Here's how the part is built. I have some questions about the finished solid (model axes, mm). Face numbers are marked on the shaded views. Coordinates: 2 decimals unless noted, no trailing zeros. Write each loop counter-clockwise with the first axis right and the second up, starting at its lowest first coordinate (ties: lowest second). Pieces come first, ordered by that corner, then holes. Notation, with made-up numbers: (74, 83) -> (117, 83) arc R30 cw to (117, 116) -> close; hole circle Ø10 at (49, -31.75). An arc over 180 degrees is marked (long way). Use a Markdown table: item, result. Add a question column.
Item 1: Will these pins go through, and if not, where does the flat tip stop? pin 1 Ø3 at (x, z) = (4, 1.5) entering from -Y; pin 2 Ø1 at (y, z) = (0.5, 7) entering from -X; pin 3 Ø3.5 at (x, z) = (0, 0) entering from +Y; pin 4 Ø1 at (x, y) = (-6, 2) entering from -Z.
Item 2: If we mould it in two halves opening along Z, with no side actions, what happens to the marked faces 1, 2, 3 and 4? For each: pulls with the +Z half, pulls with the -Z half, needs draft (parallel to the pull), parting line crosses it, or undercut.
Item 3: If I drill on line 1 along Z through (x, y) = (0, 1.25); line 2 along X through (y, z) = (1.2, 10); line 3 along Z through (x, y) = (1, 1.55), over which ranges is the centre line in solid material (lowest first)? Write a range as from..to.
Item 4: Imagine slicing it at B-B, the plane x = 0. Write out the boundary of the cut face in (y, z).
Item 5: Imagine slicing it at C-C, the plane x = -4.5. Write out the boundary of the cut face in (y, z) (3 decimals), and give its area (3 significant figures).
Item 6: Imagine slicing it at D-D, the plane y = 2.3. Count the separate pieces of the cut face and the enclosed holes in it, and give its area (3 significant figures).
Item 7: Imagine slicing it at A-A, the plane z = 0. Write out the boundary of the cut face in (x, y).
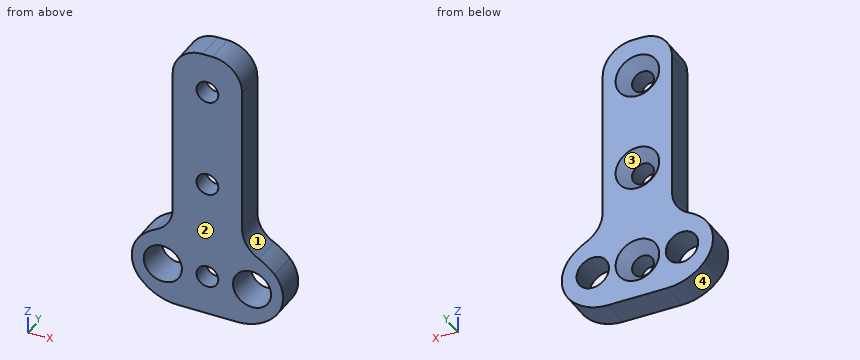
```python
from build123d import *

# Parameters (mm, degrees)
BOSS_EXTRUDE1_DEPTH                                 = 3
CSK_FOR_M2_COUNTERSUNK_FLAT_HEAD_SCREW3_D           = 2.2
CSK_FOR_M2_COUNTERSUNK_FLAT_HEAD_SCREW3_DEPTH       = 3
CSK_FOR_M2_COUNTERSUNK_FLAT_HEAD_SCREW3_CSINK_D     = 4.4
CSK_FOR_M2_COUNTERSUNK_FLAT_HEAD_SCREW3_CSINK_ANGLE = 90
CSK_FOR_M2_COUNTERSUNK_FLAT_HEAD_SCREW3_TIP         = 0.660946681
FILLET1_R                                           = 5
FILLET2_R                                           = 3.5
FILLET3_R                                           = 3
CSK_FOR_M2_COUNTERSUNK_FLAT_HEAD_SCR_2_COUNT        = 2
CSK_FOR_M2_COUNTERSUNK_FLAT_HEAD_SCR_2_PITCH        = 9


with BuildPart() as part:
    # Sketch1 → Boss-Extrude1 (new body)
    with BuildSketch(Plane(origin=(0, 0, 0), x_dir=(1, 0, 0), z_dir=(0, 1, 0))):
        Polygon((3.5, 6), (8, 6), (8, 14), (-8, 14), (-8, 6), (-3.5, 6), (-3.5, -14), (3.5, -14), align=None)
    extrude(amount=BOSS_EXTRUDE1_DEPTH)

    # CSK for M2 Countersunk Flat Head Screw3
    with Locations(Plane(origin=(0, 3, 0), x_dir=(1, 0, 0), z_dir=(0, 1, 0))):
        with Locations((0, 10), (0, 0), (0, -10)):
            CounterSinkHole(CSK_FOR_M2_COUNTERSUNK_FLAT_HEAD_SCREW3_D / 2, CSK_FOR_M2_COUNTERSUNK_FLAT_HEAD_SCREW3_CSINK_D / 2, depth=CSK_FOR_M2_COUNTERSUNK_FLAT_HEAD_SCREW3_DEPTH, counter_sink_angle=CSK_FOR_M2_COUNTERSUNK_FLAT_HEAD_SCREW3_CSINK_ANGLE)
            with Locations((0, 0, -(CSK_FOR_M2_COUNTERSUNK_FLAT_HEAD_SCREW3_DEPTH + CSK_FOR_M2_COUNTERSUNK_FLAT_HEAD_SCREW3_TIP / 2))):  # 118° drill point
                Cone(0, CSK_FOR_M2_COUNTERSUNK_FLAT_HEAD_SCREW3_D / 2, CSK_FOR_M2_COUNTERSUNK_FLAT_HEAD_SCREW3_TIP, mode=Mode.SUBTRACT)

    # Fillet1
    # the kernel refuses this fillet: 5 mm, written as the material it takes off along each edge
    with BuildSketch(Plane(origin=(-8, -12.437342964, -6), x_dir=(1, 0, 0), z_dir=(0, 1, 0))) as fillet1_piece_1:
        with BuildLine():
            CenterArc((5, 4.974937186), FILLET1_R, 180, 84.260829523)
            Line((0, 4.974937186), (-0.1, 4.974937186))
            Line((-0.1, 4.974937186), (-0.1, 0))
            Line((-0.1, 0), (0, -0.1))
            ThreePointArc((0, -0.1), (2.25, -0.1), (4.49, -0.099498744))
            Line((4.49, -0.099498744), (4.5, 0))
        make_face()
    extrude(amount=27.874685928, mode=Mode.SUBTRACT)
    with BuildSketch(Plane(origin=(-8, -12.5, -14), x_dir=(0, 0, 1), z_dir=(0, 1, 0)), Plane(origin=(8, -12.5, -14), x_dir=(-1, 0, 0), z_dir=(0, 1, 0))) as fillet1_piece_2:
        with BuildLine():
            CenterArc((FILLET1_R, FILLET1_R), FILLET1_R, 180, 90)
            Line((0, FILLET1_R), (-FILLET1_R * 0.02, FILLET1_R))
            Line((-FILLET1_R * 0.02, FILLET1_R), (-FILLET1_R * 0.02, -FILLET1_R * 0.02))
            Line((-FILLET1_R * 0.02, -FILLET1_R * 0.02), (FILLET1_R, -FILLET1_R * 0.02))
            Line((FILLET1_R, -FILLET1_R * 0.02), (FILLET1_R, 0))
        make_face()
    extrude(amount=28, mode=Mode.SUBTRACT)
    with BuildSketch(Plane(origin=(8, -12.437342964, -6), x_dir=(-1, 0, 0), z_dir=(0, 1, 0))) as fillet1_piece_3:
        with BuildLine():
            CenterArc((5, -4.974937186), FILLET1_R, 95.739170477, 84.260829523)
            Line((0, -4.974937186), (-0.1, -4.974937186))
            Line((-0.1, -4.974937186), (-0.1, 0))
            Line((-0.1, 0), (0, 0.1))
            ThreePointArc((0, 0.1), (2.25, 0.1), (4.49, 0.099498744))
            Line((4.49, 0.099498744), (4.5, 0))
        make_face()
    extrude(amount=27.874685928, mode=Mode.SUBTRACT)

    # Fillet2
    fillet2_edges = [part.edges().sort_by_distance(p)[0] for p in [
        (-7.901520762, 1.5, -9.987468593),
        (7.901520762, 1.5, -9.987468593),
    ]]
    fillet(fillet2_edges, radius=FILLET2_R)

    # Fillet3
    fillet3_edges = [part.edges().sort_by_distance(p)[0] for p in [
        (3.5, 1.5, -6),
        (3.5, 1.5, 14),
        (-3.5, 1.5, 14),
        (-3.5, 1.5, -6),
    ]]
    fillet(fillet3_edges, radius=FILLET3_R)

    # Sketch8 → CSK for M2 Countersunk Flat Head Screw2 (revolve, cut)
    with BuildSketch(Plane(origin=(-4.5, 0, -10), x_dir=(0, 0, -1), z_dir=(1, 0, 0))):
        Polygon((0, 0), (0, 3), (1.6, 3), (1.6, 3.375254051), (1.925, 0), align=None)
    csk_for_m2_countersunk_flat_head_screw2 = revolve(axis=Axis((-4.5, -6.35, -10), (0, 1, 0)), mode=Mode.SUBTRACT)

    # CSK for M2 Countersunk Flat Head Scr 2: CSK for M2 Countersunk Flat Head Screw2 ×2
    with Locations(*[(i * CSK_FOR_M2_COUNTERSUNK_FLAT_HEAD_SCR_2_PITCH, 0, 0) for i in range(1, CSK_FOR_M2_COUNTERSUNK_FLAT_HEAD_SCR_2_COUNT)]):
        add(csk_for_m2_countersunk_flat_head_screw2, mode=Mode.SUBTRACT)


solid = part.part
```
Ans:
| question | item | result |
|---|---|---|
| 1 | pin 1 | stops at y = 0 |
| 1 | pin 2 | stops at x = -3.5 |
| 1 | pin 3 | stops at y = 2.55 |
| 1 | pin 4 | stops at z = -13.33 |
| 2 | face 1 | pulls with the +Z half |
| 2 | face 2 | needs draft |
| 2 | face 3 | undercut |
| 2 | face 4 | pulls with the -Z half |
| 3 | line 1 | z = -14..-11.1, -8.9..-1.1, 1.1..8.9, 11.1..14 |
| 3 | line 2 | x = -3.5..-1.1, 1.1..3.5 |
| 3 | line 3 | z = -14..-10.46, -9.54..-0.46, 0.46..9.54, 10.46..13.96 |
| 4 | outline | (0, -14) -> (3, -14) -> (3, -12.2) -> (1.9, -11.1) -> (0, -11.1) -> close; (0, -8.9) -> (1.9, -8.9) -> (3, -7.8) -> (3, -2.2) -> (1.9, -1.1) -> (0, -1.1) -> close; (0, 1.1) -> (1.9, 1.1) -> (3, 2.2) -> (3, 7.8) -> (1.9, 8.9) -> (0, 8.9) -> close; (0, 11.1) -> (1.9, 11.1) -> (3, 12.2) -> (3, 14) -> (0, 14) -> close |
| 5 | outline | (0, -13.77) -> (3, -13.77) -> (3, -11.636) -> (0, -11.925) -> close; (0, -8.075) -> (3, -8.364) -> (3, -6.017) -> (0, -6.017) -> close |
| 5 | area | 12.6 mm^2 |
| 6 | separate pieces | 1 |
| 6 | enclosed holes | 5 |
| 6 | area | 204 mm^2 |
| 7 | outline | (-3.5, 0) -> (-1.1, 0) -> (-1.1, 1.9) -> (-2.2, 3) -> (-3.5, 3) -> close; (1.1, 0) -> (3.5, 0) -> (3.5, 3) -> (2.2, 3) -> (1.1, 1.9) -> close |
